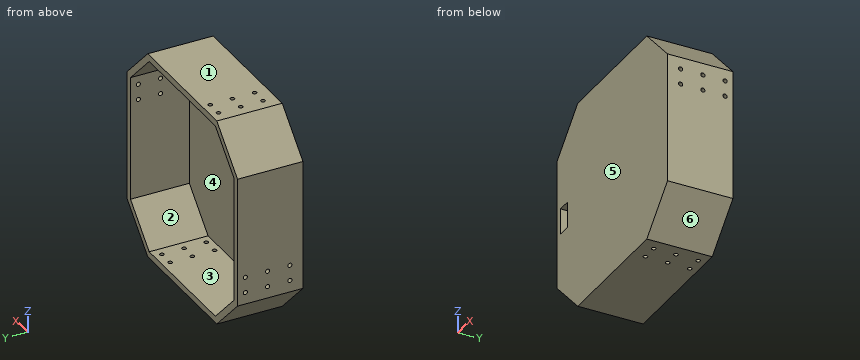
from build123d import *

# Parameters (mm, degrees)
BOSS_EXTRUDE1_DEPTH = 50
SHELL1_T            = -5
SKETCH5_W           = 10
SKETCH5_H           = 20
CUT_EXTRUDE1_DEPTH  = 5
SKETCH6_R           = 1.6
CUT_EXTRUDE2_DEPTH  = 5
CIRPATTERN1_COUNT   = 4


with BuildPart() as part:
    # Sketch1 → Boss-Extrude1 (new body)
    with BuildSketch(Plane(origin=(0, 0, 0), x_dir=(1, 0, 0), z_dir=(0, 1, 0))):
        Polygon((-50, 80), (-80, 50), (-80, -50), (-50, -80), (50, -80), (80, -50), (80, 50), (50, 80), align=None)
    extrude(amount=BOSS_EXTRUDE1_DEPTH)

    # Shell1
    shell1_openings = [part.faces().sort_by_distance(p)[0] for p in [
        (0, 50, 0),
    ]]
    offset(amount=SHELL1_T, openings=shell1_openings, kind=Kind.INTERSECTION)

    # Sketch5 → Cut-Extrude1 (cut)
    with BuildSketch(Plane(origin=(0, 5, 0), x_dir=(1, 0, 0), z_dir=(0, 1, 0))):
        with Locations((-70, 0)):
            Rectangle(SKETCH5_W, SKETCH5_H)
    extrude(amount=-CUT_EXTRUDE1_DEPTH, mode=Mode.SUBTRACT)

    # Sketch6 → Cut-Extrude2 (cut)
    with BuildSketch(Plane.XY.offset(80)):
        with Locations((-29, 10)):
            Circle(SKETCH6_R)
        with Locations((-41, 10)):
            Circle(SKETCH6_R)
        with Locations((-29, 27)):
            Circle(SKETCH6_R)
        with Locations((-41, 27)):
            Circle(SKETCH6_R)
        with Locations((-29, 44)):
            Circle(SKETCH6_R)
        with Locations((-41, 44)):
            Circle(SKETCH6_R)
    cut_extrude2 = extrude(amount=-CUT_EXTRUDE2_DEPTH, mode=Mode.SUBTRACT)

    # CirPattern1: Cut-Extrude2 ×4 about axis
    cirpattern1_axis = Axis((0, 52.5, 0), (0, -1, 0))
    for i in range(1, CIRPATTERN1_COUNT):
        add(cut_extrude2.rotate(cirpattern1_axis, i * 360 / CIRPATTERN1_COUNT), mode=Mode.SUBTRACT)


solid = part.part
Could you check a few things on this model? Use its own coordinates, in mm. Face numbers are marked on the shaded views. A direction names the side the tool comes from. Give positions to 0.01 mm unless a question says otherwise; leave off trailing zeros. Write each loop counter-clockwise with the first axis right and the second up, starting at its lowest first coordinate (ties: lowest second). Pieces come first, ordered by that corner, then holes. Notation, with made-up numbers: (-19.5, 3) -> (18.5, 3) arc R9 cw to (18.5, 11) -> close; hole circle Ø6 at (70, 9). An arc over 180 degrees is marked (long way). Write each question's results on one line, items separated by ' | '. Start each with the question number.
Q1. I need wall thicknesses on probe 1 along Y at (x, z) = (-77.5, -29); probe 2 along Z at (x, y) = (-13, 13). Which ranges of each line are inside material? Lowest first, please.
Q2. I'm going to push flat-ended pins straight in: pin 1 Ø3.5 at (y, z) = (44, 41) entering from +X; pin 2 Ø5.5 at (x, y) = (-72, 3) entering from +Z; pin 3 Ø6 at (x, y) = (-58.5, 29.5) entering from -Z; pin 4 Ø1.9 at (y, z) = (10, 29) entering from +X. Where does each tip first touch, or does it pass through?
Q3. Which directions (+Z, -Z, +X, -X, +Y, -Y) give clear straight access to the entire face, cutting with the end or side of a thin tool? Please do the marked faces 1 and 2.
Q4. Suppose I cut it at A-A, the plane z = 0. List the corners of the cut face in (x, y) for me, and give its area (3 significant figures).
Q5. Suppose I cut it at C-C, the plane x = 62. List the corners of the cut face in (y, z) for me.
Q6. Suppose I cut it at B-B, the plane y = 40.5. List the corners of the cut face in (x, z) for me.
Q7. Suppose I cut it at D-D, the plane z = 52.5. List the corners of the cut face in (x, y) for me.
Q8. We'd pull the mould along X, two halves only. Please class the marked faces 3, 4, 5 and 6: +X half, -X half, draft (parallel to the pull), parting line (faces both ways), or undercut.
Outcome:
1) probe 1: 0 to 8.4, 11.6 to 25.4, 28.6 to 42.4, 45.6 to 50 | probe 2: -80 to -75, 75 to 80
2) pin 1: x = 80 | pin 2: z = 60.75 | pin 3: z = -74.5 | pin 4: x = -75
3) face 1: +Z, +X, -X, +Y, -Y | face 2: +Y
4) outline: (-80, 0) -> (-75, 0) -> (-75, 50) -> (-80, 50) -> close; (-65, 0) -> (80, 0) -> (80, 50) -> (75, 50) -> (75, 5) -> (-65, 5) -> close | area: 1,200 mm2
5) outline: (0, -68) -> (50, -68) -> (50, -60.93) -> (5, -60.93) -> (5, 60.93) -> (50, 60.93) -> (50, 68) -> (0, 68) -> close
6) outline: (-80, -50) -> (-50, -80) -> (50, -80) -> (80, -50) -> (80, 50) -> (50, 80) -> (-50, 80) -> (-80, 50) -> close; hole (-75, -47.93) -> (-47.93, -75) -> (47.93, -75) -> (75, -47.93) -> (75, 47.93) -> (47.93, 75) -> (-47.93, 75) -> (-75, 47.93) -> close
7) outline: (-77.5, 0) -> (77.5, 0) -> (77.5, 50) -> (70.43, 50) -> (70.43, 5) -> (-70.43, 5) -> (-70.43, 50) -> (-77.5, 50) -> close
8) face 3: undercut | face 4: undercut | face 5: draft | face 6: +X half
